Geometry: see drawing. Coordinates: mm, zero at the bounding-box minimum. A direction names the side the tool comes from. Coordinates: 2 decimals unless noted, no trailing zeros. Loops run counter-clockwise (first coordinate to the right, second up) from the corner with the lowest first, then second, coordinate; pieces in that order, holes last. Notation, with made-up numbers: (84.5, -34.5) - (98.5, -34.5) arc R34 cw to (98.5, 3.5) - close; hole circle Ø10 at (21, 67.25). An arc over 180 degrees is marked (long way). Answer in a Markdown table with one row per item.
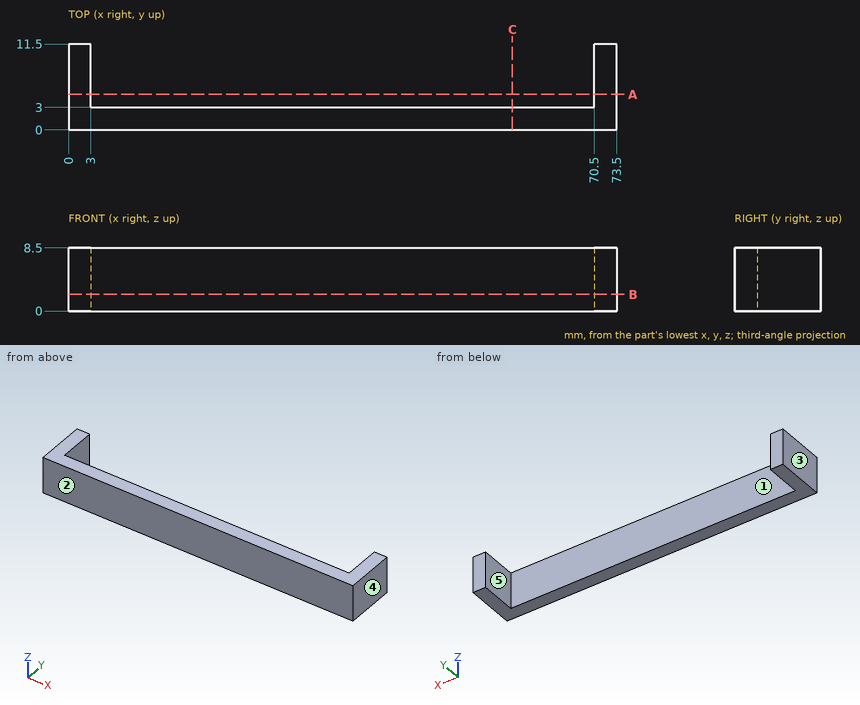
(1) Pull-direction query (X, two-part tool) for the marked faces 1, 2 and 3; classes: pulls with the +X half, pulls with the -X half, needs draft (parallel to the pull), parting line crosses it, or undercut.
Verdict:
| item | result |
|---|---|
| face 1 | undercut |
| face 2 | needs draft |
| face 3 | pulls with the -X half |
(2) Access query for the marked faces 4 and 5. Directions: +Z, -Z, +X, -X, +Y, -Y. A direction counts if a zero-diameter tool reaches every point of the face in a straight line with its end or side. Return the directions, or none.
Verdict:
| item | result |
|---|---|
| face 4 | +Z, -Z, +X, +Y, -Y |
| face 5 | +Z, -Z, +Y |
(3) Cut plane A-A on y = 4.75. Output: boundary loops of the cut face in (x, z), then the cut area to 3 significant figures.
Verdict:
| item | result |
|---|---|
| outline | (0, 0) - (3, 0) - (3, 8.5) - (0, 8.5) - close; (70.5, 0) - (73.5, 0) - (73.5, 8.5) - (70.5, 8.5) - close |
| area | 51.0 mm² |
(4) Cut plane C-C on x = 59.5. Output: boundary loops of the cut face in (y, z).
Verdict:
| item | result |
|---|---|
| outline | (0, 0) - (3, 0) - (3, 8.5) - (0, 8.5) - close |
(5) Cut plane B-B on z = 2.25. Output: boundary loops of the cut face in (x, y), then the cut area to 4 significant figures.
Verdict:
| item | result |
|---|---|
| outline | (0, 0) - (73.5, 0) - (73.5, 11.5) - (70.5, 11.5) - (70.5, 3) - (3, 3) - (3, 11.5) - (0, 11.5) - close |
| area | 271.5 mm² |
(6) Ray query, probe 1 along X at (y, z) = (5.5, 7); probe 2 along Y at (x, z) = (70, 8.25). Return the intervals inside material, ascending.
Verdict:
| item | result |
|---|---|
| probe 1 | x = 0 to 3, 70.5 to 73.5 |
| probe 2 | y = 0 to 3 |
